Read the model definition and answer for the solid it produces. Units are mm, in the model's axes. Face numbers are marked on the shaded views. A direction names the side the tool comes from. Give positions to 0.01 mm unless a question says otherwise; leave off trailing zeros. Order: outer loops, then holes, each group sorted by start corner. A loop starts at its lowest first (then second) coordinate and runs counter-clockwise, first axis right, second up. Notation, with made-up numbers: (22.25, -12) - (39.25, -12) arc R19 cw to (39.25, 10) - close; hole circle Ø3 at (22, 59). An arc over 180 degrees is marked (long way). One line per item, written item: value. Start each with the question number.
```python
from build123d import *

# Parameters (mm, degrees)
SKETCH1_R           = 26.4033
SKETCH1_R_2         = 16.8021
BOSS_EXTRUDE1_DEPTH = 31.75
SKETCH2_R           = 2.4892
BOSS_EXTRUDE2_DEPTH = 0.508


with BuildPart() as part:
    # Sketch1 → Boss-Extrude1 (new body)
    with BuildSketch(Plane.XY):
        Circle(SKETCH1_R)
        Circle(SKETCH1_R_2, mode=Mode.SUBTRACT)
    extrude(amount=BOSS_EXTRUDE1_DEPTH)

    # Sketch2 → Boss-Extrude2 (add)
    with BuildSketch(Plane(origin=(0, 25.8826, 0), x_dir=(1, 0, 0), z_dir=(0, 1, 0))):
        with BuildLine():
            Line((0, -31.75), (0, 0))
            Line((0, 0), (52.681392922, 0))
            add(Edge.make_bspline(
                [(52.681392922, -31.75), (57.642158889, -31.75), (57.642158889, -15.875), (57.642158889, 0), (52.681392922, 0)],
                knots=[3.141592654, 3.141592654, 3.141592654, 4.71238898, 4.71238898, 6.283185307, 6.283185307, 6.283185307], degree=2, weights=[1, 0.707106781, 1, 0.707106781, 1]))
            Line((52.681392922, -31.75), (0, -31.75))
        make_face()
        with Locations((52.681392922, -15.875)):
            Circle(SKETCH2_R, mode=Mode.SUBTRACT)
    extrude(amount=BOSS_EXTRUDE2_DEPTH)


solid = part.part
```
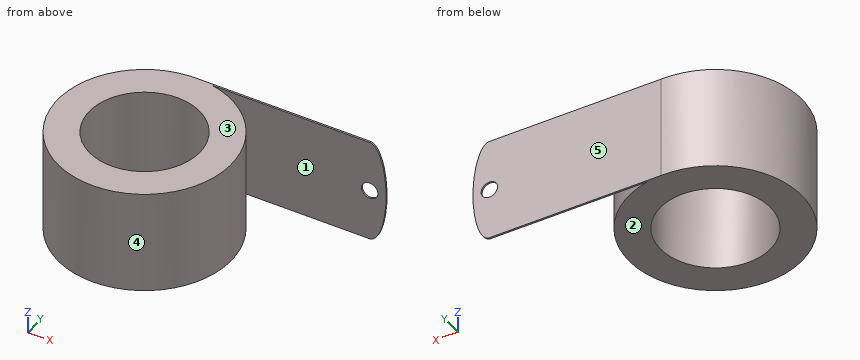
1) For the marked faces 1 and 2, determine the directions among +Z, -Z, +X, -X, +Y, -Y from which every point of the face is accessible in a straight line to the end or side of a thin tool.
2) Find the intervals of material crossed by probe 1 along Y at (x, z) = (0, 23); probe 2 along Y at (x, z) = (13.5, 20.5); probe 3 along Y at (x, z) = (14, 3), in increasing order. Write a range as from..to.
3) Each of these flat-tipped pins is pushed along its axis until it touches: pin 1 (1 mm diameter, centred on x = -3.5, z = 14.5, fed in from -Y); pin 2 (6 mm diameter, centred on x = -5.5, z = 4.5, fed in from +Y); pin 3 (1.5 mm diameter, centred on y = 19.5, z = 15.5, fed in from -X). Where does it stop, or does it pass through?
4) The mould has two halves that part along Y. Classify the marked faces 3, 4 and 5: +Y half, -Y half, draft (parallel to the pull), parting line (faces both ways), or undercut.
5) Section A-A on y = 0 is taken. Write down the section's boundary in (x, z).
6) Section C-C on y = 7.5 is taken. Write down the section's boundary in (x, z), plus the area to 3 significant figures.
7) Section B-B on z = 15 is taken. Give the number of separate pieces and of enclosed holes in the cut face, plus the area to 3 significant figures.
8) Section D-D on x = 28 is taken. Write down the section's boundary in (y, z).
Solved:
1. face 1: +Z, -Z, +X
1. face 2: -Z, +X, -X, +Y, -Y
2. probe 1: y = -26.4..-16.8, 16.8..26.4
2. probe 2: y = -22.69..-10, 10..22.69, 25.88..26.39
2. probe 3: y = -22.39..-9.29, 9.29..22.39, 25.88..26.39
3. pin 1: stops at y = -26.23
3. pin 2: stops at y = 26.28
3. pin 3: stops at x = -18.59
4. face 3: draft
4. face 4: undercut
4. face 5: +Y half
5. outline: (-26.4, 0) - (-16.8, 0) - (-16.8, 31.75) - (-26.4, 31.75) - close; (16.8, 0) - (26.4, 0) - (26.4, 31.75) - (16.8, 31.75) - close
6. outline: (-25.32, 0) - (-15.04, 0) - (-15.04, 31.75) - (-25.32, 31.75) - close; (15.04, 0) - (25.32, 0) - (25.32, 31.75) - (15.04, 31.75) - close
6. area: 653 mm2
7. separate pieces: 2
7. enclosed holes: 1
7. area: 1,330 mm2
8. outline: (25.88, 0) - (26.39, 0) - (26.39, 31.75) - (25.88, 31.75) - close
